Geometry: final body of the model. Coordinates: model frame, mm. A direction names the side the tool comes from. Coordinates: 2 decimals unless noted, no trailing zeros. Loops run counter-clockwise (first coordinate to the right, second up) from the corner with the lowest first, then second, coordinate; pieces in that order, holes last. Notation, with made-up numbers: (80, 32.5) - (120, 32.5) arc R26 cw to (120, 63.5) - close; hole circle Ø5 at (-7.5, -14). An arc over 180 degrees is marked (long way). Answer in a Markdown table with one row per item.
from build123d import *

# Parameters (mm, degrees)
F0_R      = 45
F1_DEPTH  = 3
F4_R      = 5.08
F5_R      = 26
F6_DEPTH  = 37.8739
F6_TAPER  = -3
F9_R      = 36
F10_DEPTH = 6.894


with BuildPart() as f1:
    # F0 (on Top) → F1 (new body)
    with BuildSketch(Plane.XY):
        Circle(F0_R)
    extrude(amount=F1_DEPTH)

    # F2 (on Front) → F3 (revolve)
    with BuildSketch(Plane.XZ):
        Polygon((-40.5863100491, 0), (0, 0), (0, 24.3678710608), (-35, 24.3678710608), align=None)
    revolve(axis=Axis((0, 0, -19.3198865833), (0, 0, -1)))

    # F4
    f4_edges = [f1.edges().sort_by_distance(p)[0] for p in [
        (35, 0, 24.367871),
    ]]
    fillet(f4_edges, radius=F4_R)

    # F5 (on Top) → F6 (cut, symmetric)
    with BuildSketch(Plane.XY):
        Circle(F5_R)
    extrude(amount=F6_DEPTH, both=True, taper=F6_TAPER, mode=Mode.SUBTRACT)

    # F7 (on Front) → F8 (revolve, cut)
    with BuildSketch(Plane.XZ):
        Polygon((35.8599051833, 18.4277258813), (30.9155862778, 18.4277258813), (20.1216544956, 0), (26.0245222598, 0), (31.2158084296, 13.110072352), (35.8599051833, 13.110072352), align=None)
    revolve(axis=Axis((0, 0, 14.1704455018), (0, 0, -1)), mode=Mode.SUBTRACT)

    # F9 (on face) → F10 (cut)
    with BuildSketch(Plane(origin=(0, 0, 0), x_dir=(1, 0, 0), z_dir=(0, 0, -1))):
        Circle(F9_R)
    extrude(amount=-F10_DEPTH, mode=Mode.SUBTRACT)


solid = f1.part
(1) Access query for faces 1 (the face through (-21.26, 16.3, 11.38)), 2 (the face through (2.1, -27.4, 24.368)), 3 (the face through (-4.686, -35.694, 3.399)). Directions: +Z, -Z, +X, -X, +Y, -Y. A direction counts if a zero-diameter tool reaches every point of the face in a straight line with its end or side. Return the directions, or none.
Verdict:
| item | result |
|---|---|
| face 1 | none |
| face 2 | +Z, +X, -X, +Y, -Y |
| face 3 | -Z |
(2) First-contact query: pin 1 Ø1.5 at (x, z) = (25, 10) entering from +Y; pin 2 Ø1.5 at (y, z) = (16, 20.5) entering from +X; pin 3 Ø4 at (y, z) = (-2.5, 15.5) entering from -X. Flat tips, straight axial feed; report the tip coordinate or a pass-through.
Verdict:
| item | result |
|---|---|
| pin 1 | stops at y = 29.68 |
| pin 2 | stops at x = 32.53 |
| pin 3 | stops at x = -37.42 |
(3) Pull-direction query (X, two-part tool) for faces 4 (the face through (-2, -32, 13.11)), 5 (the face through (-5.822, -26.216, 16.305)), 6 (the face through (-16.683, -32.075, 19.333)), 7 (the face through (-4, -40, 3)); classes: pulls with the +X half, pulls with the -X half, needs draft (parallel to the pull), parting line crosses it, or undercut.
Verdict:
| item | result |
|---|---|
| face 4 | undercut |
| face 5 | undercut |
| face 6 | parting line crosses it |
| face 7 | needs draft |
(4) Cut plane A-A on x = 0. Output: boundary loops of the cut face in (y, z), then the cut area to 3 significant figures.
Verdict:
| item | result |
|---|---|
| outline | (-45, 0) - (-36, 0) - (-36, 6.89) - (-28.75, 6.89) - (-31.22, 13.11) - (-35.86, 13.11) - (-35.86, 18.43) - (-30.92, 18.43) - (-26.58, 11.02) - (-27.28, 24.37) - (-30.95, 24.37) arc R5.08 ccw to (-35.9, 20.42) - (-39.9, 3) - (-45, 3) - close; (26.58, 11.02) - (30.92, 18.43) - (35.86, 18.43) - (35.86, 13.11) - (31.22, 13.11) - (28.75, 6.89) - (36, 6.89) - (36, 0) - (45, 0) - (45, 3) - (39.9, 3) - (35.9, 20.42) arc R5.08 ccw to (30.95, 24.37) - (27.28, 24.37) - close |
| area | 321 mm² |
(5) Ray query, probe 1 along Y at (x, z) = (0, 16.1); probe 2 along X at (y, z) = (-11, 17.25); probe 3 along Z at (x, y) = (-32, 28.5). Return the intervals inside material, ascending.
Verdict:
| item | result |
|---|---|
| probe 1 | y = -36.9 to -35.86, -29.55 to -26.84, 26.84 to 29.55, 35.86 to 36.9 |
| probe 2 | x = -34.94 to -34.13, -28.15 to -24.55, 24.55 to 28.15, 34.13 to 34.94 |
| probe 3 | z = 0 to 3 |
